from build123d import *

# Parameters (mm, degrees)
F0_R     = 1.5875
F1_DEPTH = 3.175
F2_W     = 5.0304289907
F2_H     = 4.9511287361
F3_DEPTH = 0.762
F4_W     = 5.1232710698
F4_H     = 5.2371935268
F5_DEPTH = 0.508
F6_W     = 0.5395373363
F6_H     = 6.858
F7_DEPTH = 0.889


with BuildPart() as f1:
    # F0 (on Front) → F1 (new body)
    with BuildSketch(Plane.XZ):
        with Locations((-24.2014154792, 23.8942243159)):
            Circle(F0_R)
    extrude(amount=F1_DEPTH)

    # F2 (on Front) → F3 (join)
    with BuildSketch(Plane.XZ):
        with Locations((-24.3402747437, 24.8939255252)):
            Rectangle(F2_W, F2_H)
    extrude(amount=-F3_DEPTH)

    # F4 (on face) → F5 (join)
    with BuildSketch(Plane(origin=(0, 0, 22.4183611572), x_dir=(1, 0, 0), z_dir=(0, 0, -1))):
        with Locations((-24.3866957833, -3.3805967634)):
            Rectangle(F4_W, F4_H)
    extrude(amount=-F5_DEPTH)

    # F6 (on face) → F7 (join)
    with BuildSketch(Plane(origin=(0, 0, 22.4183611572), x_dir=(1, 0, 0), z_dir=(0, 0, -1))):
        with Locations((-24.1154753933, -2.9085015029)):
            Rectangle(F6_W, F6_H)
    extrude(amount=F7_DEPTH)


solid = f1.part
For this review, take the finished solid that the model builds, in its own axes (mm). A direction names the side the tool comes from. Round coordinates to 2 decimals unless told otherwise and drop trailing zeros. Order: outer loops, then holes, each group sorted by start corner. A loop starts at its lowest first (then second) coordinate and runs counter-clockwise, first axis right, second up. Notation, with made-up numbers: M 49,-32 L 55,-32 A10 ccw 55,-25 Z; hole C 57,77 d11. An arc over 180 degrees is marked long. Use a Markdown table: item, result. Add a question column.
Item 1: Add section C-C, the plane x = -22.35. Give the boundary of the cut face in (y, z), then the cut area to 3 significant figures.
Item 2: To check wall thickness, follow line 1 along Z through (x, y) = (-23.8, 5.25); line 2 along X through (y, z) = (3, 22.35); line 3 along Y through (x, z) = (-25.35, 25.6). State the ranges of each line that lie inside material, in increasing order.
Item 3: Add section B-B, the plane z = 23.2. Give the boundary of the cut face in (x, y) (3 decimals), then the cut area to 3 significant figures.
Item 4: Add section A-A, the plane y = 0.5. Give the boundary of the cut face in (x, z), then the cut area to 3 significant figures.
Item 5: Tool access review of faces 1 (the flat face through (-24, 3, 22.926)), 2 (the flat face through (-21.825, 1.7, 22.7)), 3 (the cylindrical face through (-24.546, -1.565, 22.344)): name each direction out of +Z, -Z, +X, -X, +Y, -Y from which nothing blocks a thin tool from reaching the whole face with its end or side.
Item 6: Insertion check: pin 1 (1.5 mm diameter, centred on x = -26, z = 26, fed in from -Y); pin 2 (2 mm diameter, centred on x = -25, z = 25, fed in from +Y); pin 3 (1 mm diameter, centred on x = -25.5, z = 22.5, fed in from +Y); pin 4 (2 mm diameter, centred on x = -24.5, y = 2.5, fed in from -Z). Each pin has a flat end and moves straight along its axis. Give the tip position at first contact, or say it passes through.
Geometry results:
| question | item | result |
|---|---|---|
| 1 | outline | M 0,22.42 L 6,22.42 L 6,22.93 L 0.76,22.93 L 0.76,27.37 L 0,27.37 Z |
| 1 | area | 6.43 mm² |
| 2 | line 1 | z = 22.42 to 22.93 |
| 2 | line 2 | x = -24.39 to -23.85 |
| 2 | line 3 | y = 0 to 0.76 |
| 3 | outline | M -26.855,0 L -25.629,0 L -25.629,-3.175 L -22.774,-3.175 L -22.774,0 L -21.825,0 L -21.825,0.762 L -26.855,0.762 Z |
| 3 | area | 12.9 mm² |
| 4 | outline | M -26.86,22.42 L -24.39,22.42 L -24.39,21.53 L -23.85,21.53 L -23.85,22.42 L -21.83,22.42 L -21.83,27.37 L -26.86,27.37 Z |
| 4 | area | 25.4 mm² |
| 5 | face 1 | +Z, +X, -X, +Y |
| 5 | face 2 | +Z, -Z, +X, +Y, -Y |
| 5 | face 3 | -Y |
| 6 | pin 1 | stops at y = 0 |
| 6 | pin 2 | stops at y = 0.76 |
| 6 | pin 3 | stops at y = 6 |
| 6 | pin 4 | stops at z = 21.53 |
